Print and shaded views of the part. All mm, measured from the part's lowest x, y and z. Coordinates: 2 decimals unless noted, no trailing zeros. Order: outer loops, then holes, each group sorted by start corner. A loop starts at its lowest first (then second) coordinate and runs counter-clockwise, first axis right, second up.
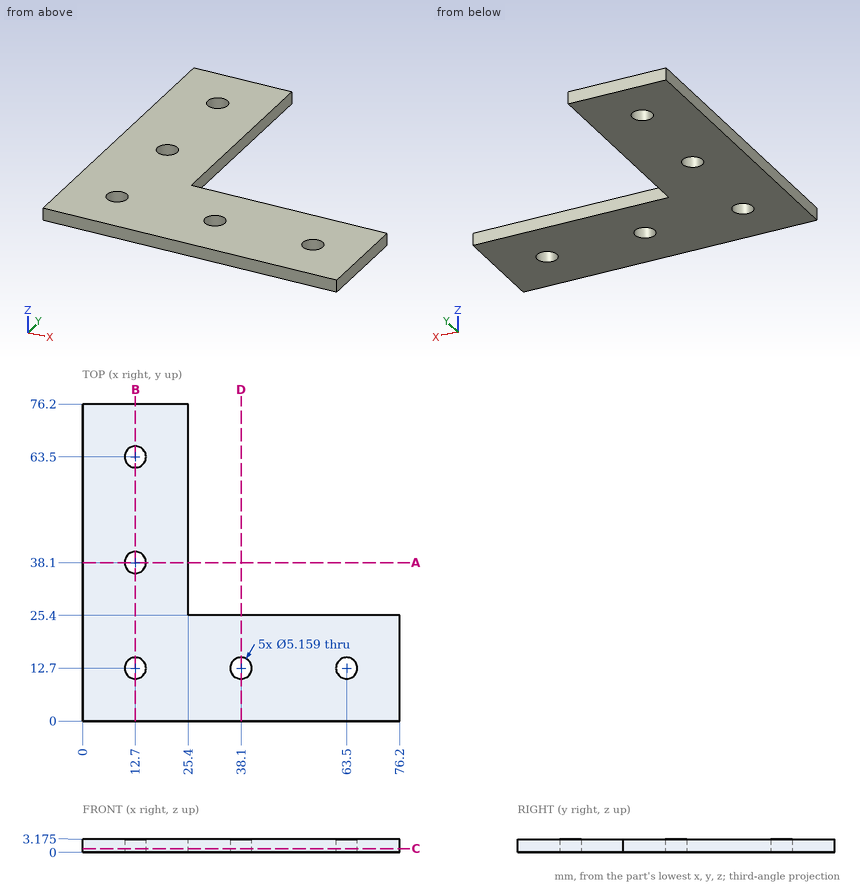
Q1. Cut at C-C, the plane z = 0.85. List the corners of the cut face in (x, y), plus the area to 3 significant figures.
Established:
outline: (0, 0) - (76.2, 0) - (76.2, 25.4) - (25.4, 25.4) - (25.4, 76.2) - (0, 76.2) - close; hole circle Ø5.16 at (12.7, 12.7); hole circle Ø5.16 at (12.7, 38.1); hole circle Ø5.16 at (12.7, 63.5); hole circle Ø5.16 at (38.1, 12.7); hole circle Ø5.16 at (63.5, 12.7)
area: 3,120 mm2
Q2. Cut at A-A, the plane y = 38.1. List the corners of the cut face in (x, z) (1 decimal).
Established:
outline: (0, 0) - (10.1, 0) - (10.1, 3.2) - (0, 3.2) - close; (15.3, 0) - (25.4, 0) - (25.4, 3.2) - (15.3, 3.2) - close
Q3. Probe line 1 (X direction, y = 13, z = 2.5); line 2 (Y direction, x = 12.7, z = 2.3); line 3 (Y direction, x = 63.5, z = 1.65). List the from-to ranges inside material, lowest first.
Established:
line 1: x = 0 to 10.14, 15.26 to 35.54, 40.66 to 60.94, 66.06 to 76.2
line 2: y = 0 to 10.12, 15.28 to 35.52, 40.68 to 60.92, 66.08 to 76.2
line 3: y = 0 to 10.12, 15.28 to 25.4
Q4. Drop flat-ended pins along their axis: P1, Ø1.5, axis at y = 28.5, z = 1.5, coming from the +X side; P2, Ø3, axis at x = 63.5, y = 12.7, coming from the +Z side. Give the stop position or say it passes through.
Established:
P1: stops at x = 25.4
P2: passes through
Q5. Cut at B-B, the plane x = 12.7. List the corners of the cut face in (y, z) (1 decimal).
Established:
outline: (0, 0) - (10.1, 0) - (10.1, 3.2) - (0, 3.2) - close; (15.3, 0) - (35.5, 0) - (35.5, 3.2) - (15.3, 3.2) - close; (40.7, 0) - (60.9, 0) - (60.9, 3.2) - (40.7, 3.2) - close; (66.1, 0) - (76.2, 0) - (76.2, 3.2) - (66.1, 3.2) - close
